The listing builds one solid part. Answer for the finished solid, in the listing's coordinates (mm). Give positions to 0.01 mm unless a question says otherwise; leave off trailing zeros. Order: outer loops, then holes, each group sorted by start corner. A loop starts at its lowest first (then second) coordinate and runs counter-clockwise, first axis right, second up. Notation, with made-up numbers: M 39.25,-28 L 59.25,-28 A35 cw 59.25,7 Z; hole C 8.5,40 d4. An arc over 180 degrees is marked long. Answer as a JSON object with one key per item and string values. Group by question number.
```python
from build123d import *

# Parameters (mm, degrees)
SKETCH_1_R          = 1
EXTRUDE_1_DEPTH     = 3.5
SKETCH_2_R          = 2
CUT_EXTRUDE_1_DEPTH = 97.753552906


with BuildPart() as part:
    # Эскиз1 → Вытянуть1 (new body)
    with BuildSketch(Plane(origin=(0, 0, 0), x_dir=(1, 0, 0), z_dir=(0, 1, 0))):
        with BuildLine():
            Line((-15, 80), (-17.987249423, 0.677390733))
            ThreePointArc((-17.987249423, 0.677390733), (0, -18), (17.987249423, 0.677390733))
            Line((17.987249423, 0.677390733), (15, 80))
            ThreePointArc((15, 80), (0, 95), (-15, 80))
        make_face()
        with Locations(Location((0, 0, 0), (0, 0, 270))):
            Circle(SKETCH_1_R, mode=Mode.SUBTRACT)
    extrude(amount=EXTRUDE_1_DEPTH)

    # Эскиз2 → Вырез-Вытянуть1 (cut, through all)
    with BuildSketch(Plane.XZ):
        with Locations(Location((-0.408986403, 12.99356495, 0), (0, 0, 270))):
            Circle(SKETCH_2_R)
        with Locations(Location((-9.477034947, 8.898640829, 0), (0, 0, 270))):
            Circle(SKETCH_2_R)
        with Locations(Location((8.898640829, 9.477034947, 0), (0, 0, 270))):
            Circle(SKETCH_2_R)
        with Locations(Location((9.477034947, -8.898640829, 0), (0, 0, 270))):
            Circle(SKETCH_2_R)
        with Locations(Location((0.408986403, -12.99356495, 0), (0, 0, 270))):
            Circle(SKETCH_2_R)
        with Locations(Location((-8.898640829, -9.477034947, 0), (0, 0, 270))):
            Circle(SKETCH_2_R)
    extrude(amount=-CUT_EXTRUDE_1_DEPTH, mode=Mode.SUBTRACT)


solid = part.part
```
Item 1: Section A-A (y = 0.7) is taken. Determine the outline of the cut face in (x, z), and give its area (3 significant figures).
Item 2: Section C-C (x = 14) is taken. Determine the outline of the cut face in (y, z), and give its area (3 significant figures).
Item 3: Section B-B (z = -29) is taken. Determine the outline of the cut face in (x, y), and give its area (3 significant figures).
Item 4: Consider probe 1 along Z at (x, y) = (10, 1.7); probe 2 along X at (y, z) = (1.35, 0); probe 3 along Z at (x, y) = (8, 1.35). Determine where each line is inside the solid, lowest interval first. Write a range as from..to.
Item 5: Determine the mould class of faces 1 (the flat face through (0, 3.5, -39)), 2 (the cylindrical face through (0, 2, -95)), 3 (the cylindrical face through (-9.665, 1.726, -11.325)), 4 (the cylindrical face through (11.46, 1.73, -8.64)) for opening direction Z: released by +Z, released by -Z, zero draft, split by the parting line, or undercut.
Item 6: Flat-ended cylindrical pins translate along their axes: P1, Ø1, axis at y = 3, z = -82.5, coming from the +X side; P2, Ø2.5, axis at x = -9.48, z = 8.9, coming from the +Y side. Find the tip coordinate at first contact, or state that the pin passes through.
Values found:
{
 "1": {"outline": "M -17.99,-0.68 L -15,-80 A15 ccw 15,-80 L 17.99,-0.68 A18 ccw long Z; hole C -9.48,8.9 d4; hole C -8.9,-9.48 d4; hole C -0.41,12.99 d4; hole C 0.41,-12.99 d4; hole C 0,0 d2; hole C 8.9,9.48 d4; hole C 9.48,-8.9 d4", "area": "3,420 mm^2"},
 "2": {"outline": "M 0,-85.39 L 3.5,-85.39 L 3.5,11.31 L 0,11.31 Z", "area": "338 mm^2"},
 "3": {"outline": "M -16.92,0 L 16.92,0 L 16.92,3.5 L -16.92,3.5 Z", "area": "118 mm^2"},
 "4": {"probe 1": "z = -91.18..-10.83, -6.97..7.81, 11.15..14.97", "probe 2": "x = -18..-1, 1..18", "probe 3": "z = -92.69..-10.25, -7.55..7.69, 11.26..16.12"},
 "5": {"face 1": "zero draft", "face 2": "released by -Z", "face 3": "undercut", "face 4": "undercut"},
 "6": {"P1": "stops at x = 14.87", "P2": "passes through"}
}
